from build123d import *

# Parameters (mm, degrees)
CROQUIS1_R                   = 25.4
SALIENTE_EXTRUIR1_DEPTH      = 12.7
SALIENTE_EXTRUIR2_REACH      = 73.887
SALIENTE_EXTRUIR2_END_RADIUS = 25.4
CROQUIS2_R                   = 12.7
CROQUIS6_R                   = 6.35
SALIENTE_EXTRUIR5_DEPTH      = 34.29


with BuildPart() as part:
    # Croquis1 → Saliente-Extruir1 (new, symmetric)
    with BuildSketch(Plane(origin=(0, 0, 0), x_dir=(0, 0, -1), z_dir=(1, 0, 0))):
        Circle(CROQUIS1_R)
    extrude(amount=SALIENTE_EXTRUIR1_DEPTH, both=True)

    # Saliente-Extruir2: up to this cylinder (the profile starts outside it)
    saliente_extruir2_end = Plane(origin=(0, 0, 0), z_dir=(-1, 0, 0)) * Cylinder(SALIENTE_EXTRUIR2_END_RADIUS, 199.574, mode=Mode.PRIVATE)
    # Croquis2 → Saliente-Extruir2 (add, up to the surface)
    with BuildSketch(Plane.XY.offset(40.64), mode=Mode.PRIVATE) as saliente_extruir2_sk1:
        Circle(CROQUIS2_R)
    saliente_extruir2_tool1 = extrude(saliente_extruir2_sk1.sketch, amount=-SALIENTE_EXTRUIR2_REACH, mode=Mode.PRIVATE) - saliente_extruir2_end
    add(saliente_extruir2_tool1.solids().sort_by_distance((0, 0, 40.64))[0])

    # Croquis6 → Saliente-Extruir5 (add, symmetric)
    with BuildSketch(Plane(origin=(0, 0, 0), x_dir=(0, 0, -1), z_dir=(1, 0, 0))):
        Circle(CROQUIS6_R)
    extrude(amount=SALIENTE_EXTRUIR5_DEPTH, both=True)


solid = part.part
For this review, take the finished solid that the model builds, in its own axes (mm). A direction names the side the tool comes from. Give positions to 0.01 mm unless a question says otherwise; leave off trailing zeros. Order: outer loops, then holes, each group sorted by start corner. A loop starts at its lowest first (then second) coordinate and runs counter-clockwise, first axis right, second up. Notation, with made-up numbers: M -13.75,-4.5 L 15.25,-4.5 A24 ccw 15.25,34.5 Z; hole C 13.5,42.25 d11. An arc over 180 degrees is marked long. Answer in a Markdown table with one row per item. Add a question column.
(1) Consider section B-B on x = 0. State the section outline as (y, z) points.
(2) Wall thickness on probe 1 along X at (y, z) = (11, 5); probe 2 along Y at (x, z) = (-1.5, -22); probe 3 along Z at (x, y) = (-19.5, 0.5): over which ranges is each line inside the solid? List them lowest first. Write a range as [from, to].
(3) Consider section D-D on x = -30. State the section outline as (y, z) points.
(4) For pin 1 (12 mm diameter, centred on x = 25, z = -2.5, fed in from -Y); pin 2 (2 mm diameter, centred on x = 14.5, z = 20.5, fed in from +Y); pin 3 (12 mm diameter, centred on y = -20, z = 0, fed in from -X); pin 4 (3 mm diameter, centred on x = -21, y = -3, fed in from -Z), all flat-tipped, find the tip position at first contact; note any pin that passes through.
(5) Consider section A-A on z = 0. State the section outline as (x, y) points, and give its area (3 significant figures).
(6) For faces 1 (the face through (-23.34, -6.2, 1.38)), 2 (the face through (12.114, 3.815, 31.449)), 3 (the face through (-34.29, 0, 0)), 4 (the face through (23.65, -6.2, 1.38)), list the 3-axis set-ups (+Z, -Z, +X, -X, +Y, -Y) from which the entire face can be reached by the end or side of a thin tool; tool diameter is ignored.
(7) Consider section C-C on y = -9. State the section outline as (x, z) points.
Evaluation:
| question | item | result |
|---|---|---|
| 1 | outline | M -12.7,22 A25.4 ccw long 12.7,22 L 12.7,40.64 L -12.7,40.64 Z |
| 2 | probe 1 | x = [-12.7, 12.7] |
| 2 | probe 2 | y = [-12.69, 12.69] |
| 2 | probe 3 | z = [-6.33, 6.33] |
| 3 | outline | C 0,0 d12.7 |
| 4 | pin 1 | stops at y = -6.35 |
| 4 | pin 2 | passes through |
| 4 | pin 3 | stops at x = -12.7 |
| 4 | pin 4 | stops at z = -6.17 |
| 5 | outline | M -34.29,-6.35 L -12.7,-6.35 L -12.7,-25.4 L 12.7,-25.4 L 12.7,-6.35 L 34.29,-6.35 L 34.29,6.35 L 12.7,6.35 L 12.7,25.4 L -12.7,25.4 L -12.7,6.35 L -34.29,6.35 Z |
| 5 | area | 1,840 mm^2 |
| 6 | face 1 | -X |
| 6 | face 2 | +Z |
| 6 | face 3 | +Z, -Z, -X, +Y, -Y |
| 6 | face 4 | +X |
| 7 | outline | M -12.7,-23.75 L 12.7,-23.75 L 12.7,23.75 L 8.96,23.75 L 8.96,40.64 L -8.96,40.64 L -8.96,23.75 L -12.7,23.75 Z |
